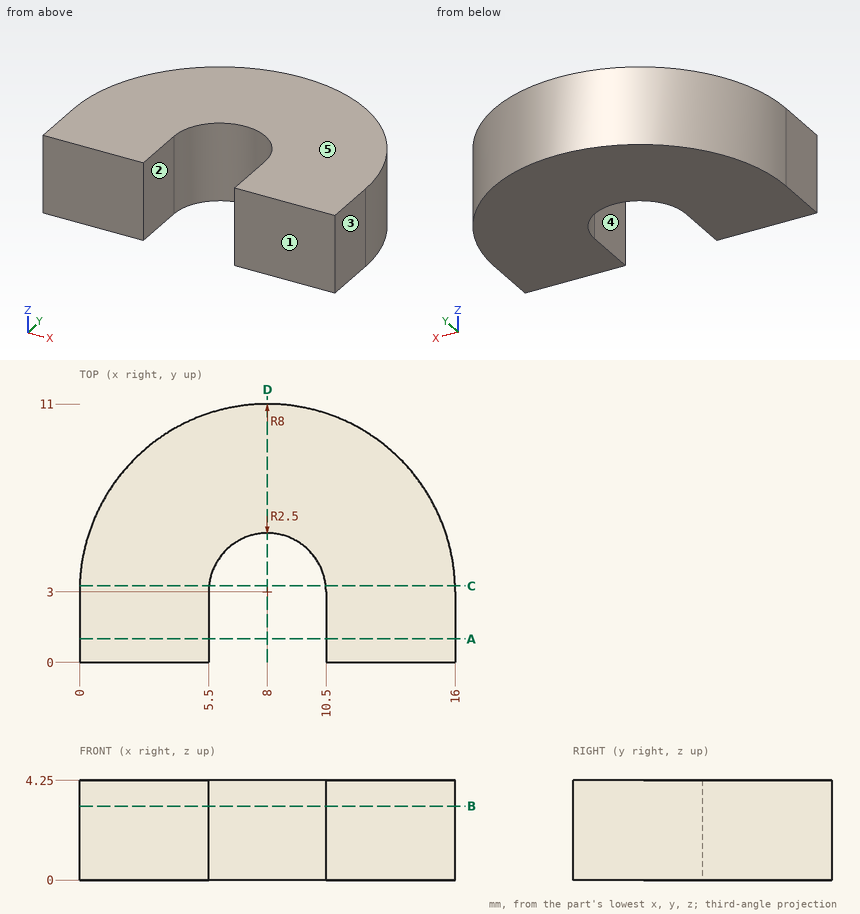
Here's the drawing with two shaded views (mm, measured from the low corner). I have some questions. A direction names the side the tool comes from. Give positions to 0.01 mm unless a question says otherwise; leave off trailing zeros. Order: outer loops, then holes, each group sorted by start corner. A loop starts at its lowest first (then second) coordinate and runs counter-clockwise, first axis right, second up. Notation, with made-up numbers: (-34.75, -30.75) - (9.25, -30.75) arc R24 cw to (9.25, -2.75) - close; hole circle Ø8 at (45.5, 47.5). An arc over 180 degrees is marked (long way). Use a Markdown table: item, result. Add a question column.
Q1. If we section it at A-A on y = 1: Write out the boundary of the cut face in (x, z), plus the area to 4 significant figures.
Q2. If we section it at C-C on y = 3.25: Write out the boundary of the cut face in (x, z), plus the area to 3 significant figures.
Q3. If we mould it in two halves opening along X, with no side actions, what happens to the marked faces 1, 2 and 3? For each: released by +X, released by -X, zero draft, split by the parting line, or undercut.
Q4. If we section it at B-B on z = 3.15: Write out the boundary of the cut face in (x, y).
Q5. On a 3-axis mill with a long thin cutter (end or side, diameter ignored), from which of +Z, -Z, +X, -X, +Y, -Y can I reach the whole of each face in a straight line? I mean the marked faces 4 and 5. Say none if no direction works.
Q6. I'm going to push flat-ended pins straight in: pin 1 (1 mm diameter, centred on x = 7.5, y = 2.5, fed in from -Z) (1 decimal); pin 2 (1.5 mm diameter, centred on x = 13.5, z = 2, fed in from -Y). Where does each tip first touch, or does it pass through?
Q7. If we section it at D-D on x = 8: Write out the boundary of the cut face in (y, z), plus the area to 3 significant figures.
Q8. Please list where these lines run through material, in increasing order: line 1 along X through (y, z) = (2.5, 3.4); line 2 along Y through (x, z) = (8, 2.95); line 3 along X through (y, z) = (4.5, 1.05).
Answers follow:
| question | item | result |
|---|---|---|
| 1 | outline | (0, 0) - (5.5, 0) - (5.5, 4.25) - (0, 4.25) - close; (10.5, 0) - (16, 0) - (16, 4.25) - (10.5, 4.25) - close |
| 1 | area | 46.75 mm^2 |
| 2 | outline | (0, 0) - (5.51, 0) - (5.51, 4.25) - (0, 4.25) - close; (10.49, 0) - (16, 0) - (16, 4.25) - (10.49, 4.25) - close |
| 2 | area | 46.8 mm^2 |
| 3 | face 1 | zero draft |
| 3 | face 2 | undercut |
| 3 | face 3 | released by +X |
| 4 | outline | (0, 0) - (5.5, 0) - (5.5, 3) arc R2.5 cw to (10.5, 3) - (10.5, 0) - (16, 0) - (16, 3) arc R8 ccw to (0, 3) - close |
| 5 | face 4 | +Z, -Z, -Y |
| 5 | face 5 | +Z, +X, -X, +Y, -Y |
| 6 | pin 1 | passes through |
| 6 | pin 2 | stops at y = 0 |
| 7 | outline | (5.5, 0) - (11, 0) - (11, 4.25) - (5.5, 4.25) - close |
| 7 | area | 23.4 mm^2 |
| 8 | line 1 | x = 0 to 5.5, 10.5 to 16 |
| 8 | line 2 | y = 5.5 to 11 |
| 8 | line 3 | x = 0.14 to 6, 10 to 15.86 |
